from build123d import *

# Parameters (mm, degrees)
BOSS_EXTRU_1_DEPTH         = 3
BOSS_EXTRU_2_DEPTH         = 100
R_P_TITION_LIN_AIRE1_COUNT = 2
R_P_TITION_LIN_AIRE1_PITCH = 103
ESQUISSE5_W                = 2.97567345
ESQUISSE5_H                = 100
BOSS_EXTRU_3_DEPTH         = 47
ESQUISSE6_W                = 2.99565123
ESQUISSE6_H                = 100
ENL_V_MAT_EXTRU_1_REACH    = 125.839
ESQUISSE7_W                = 30
ESQUISSE7_H                = 20
ESQUISSE9_R                = 1.462141601
ENL_V_MAT_EXTRU_8_DEPTH    = 10


with BuildPart() as part:
    # Esquisse2 → Boss.-Extru.1 (new body)
    with BuildSketch(Plane.XY):
        Polygon((0, 0), (0, 50), (3.942801894, 50), (37.89429856, 28.942702884), (30, 0), align=None)
    boss_extru_1 = extrude(amount=BOSS_EXTRU_1_DEPTH)

    # Esquisse4 → Boss.-Extru.2 (add)
    with BuildSketch(Plane.XY.offset(3)):
        Polygon((0, 0), (0, 3.006117571), (30.819936884, 3.006117571), (30, 0), align=None)
    extrude(amount=BOSS_EXTRU_2_DEPTH)

    # Répétition linéaire1: Boss.-Extru.1 ×2
    with Locations(*[(0, 0, i * R_P_TITION_LIN_AIRE1_PITCH) for i in range(1, R_P_TITION_LIN_AIRE1_COUNT)]):
        add(boss_extru_1)

    # Esquisse5 → Boss.-Extru.3 (add)
    with BuildSketch(Plane(origin=(0, 3.006117571, 0), x_dir=(1, 0, 0), z_dir=(0, 1, 0))):
        with Locations((1.487836725, -53)):
            Rectangle(ESQUISSE5_W, ESQUISSE5_H)
    extrude(amount=BOSS_EXTRU_3_DEPTH)

    # Balayage1: sweep along a curve in space
    with BuildLine() as balayage1_path:
        Line((30.819936884, 3.006117571, 103), (37.89429856, 28.942702884, 103))
    # Esquisse6 → Balayage1 (sweep)
    with BuildSketch(Plane(origin=(0, 3.006117571, 0), x_dir=(1, 0, 0), z_dir=(0, 1, 0))):
        with Locations((29.322111269, -53)):
            Rectangle(ESQUISSE6_W, ESQUISSE6_H)
    sweep(path=balayage1_path.line)

    # Esquisse7 → Enlèv. mat.-Extru.1 (cut, up to next)
    with BuildSketch(Plane(origin=(27.922668341, -7.616077924, 0), x_dir=(0, 0, -1), z_dir=(0.9647567628041306, -0.2631432853479158, 0)), mode=Mode.PRIVATE) as enl_v_mat_extru_1_sk1:
        with Locations((-78, 22.89429856)):
            Rectangle(ESQUISSE7_W, ESQUISSE7_H)
    enl_v_mat_extru_1_tool1 = extrude(enl_v_mat_extru_1_sk1.sketch, amount=-ENL_V_MAT_EXTRU_1_REACH, mode=Mode.PRIVATE) & part.part
    enl_v_mat_extru_1 = enl_v_mat_extru_1_tool1.solids().sort_by_distance((33.947149, 14.471351, 78))[0]
    add(enl_v_mat_extru_1, mode=Mode.SUBTRACT)

    # Symétrie1: Enlèv. mat.-Extru.1 across plane
    add(enl_v_mat_extru_1.mirror(Plane.XY.offset(53)), mode=Mode.SUBTRACT)

    # Esquisse9 → Enlèv. mat.-Extru.8 (cut)
    with BuildSketch(Plane(origin=(2.97567345, 0, 0), x_dir=(0, 0, -1), z_dir=(1, 0, 0))):
        with Locations((-84.107906361, 18.157522719)):
            Circle(ESQUISSE9_R)
    enl_v_mat_extru_8 = extrude(amount=-ENL_V_MAT_EXTRU_8_DEPTH, mode=Mode.SUBTRACT)

    # Symétrie3: Enlèv. mat.-Extru.8 across plane
    add(enl_v_mat_extru_8.mirror(Plane.XY.offset(53)), mode=Mode.SUBTRACT)


solid = part.part
The model under review builds one solid part; all positions refer to its coordinate system, in mm. A direction names the side the tool comes from. Coordinates: 2 decimals unless noted, no trailing zeros. Order: outer loops, then holes, each group sorted by start corner. A loop starts at its lowest first (then second) coordinate and runs counter-clockwise, first axis right, second up. Notation, with made-up numbers: (-40, 44) -> (-12, 44) arc R8 ccw to (-12, 49) -> close; hole circle Ø10 at (17, -12.75). An arc over 180 degrees is marked (long way). Answer in a Markdown table with one row per item.
(1) Wall thickness on line 1 along Z through (x, y) = (29, 5.5); line 2 along Z through (x, y) = (28.5, 17); line 3 along Y through (x, z) = (24, 11.5): over which ranges is each line inside the solid? List them lowest first.
Answers:
| item | result |
|---|---|
| line 1 | 0 to 13, 43 to 63, 93 to 106 |
| line 2 | 0 to 3, 103 to 106 |
| line 3 | 0 to 3.01 |
(2) Consider section D-D (x = 7.5). Write out the cut boundary in (y, z), plus the area to 3 significant figures.
Answers:
| item | result |
|---|---|
| outline | (0, 0) -> (47.79, 0) -> (47.79, 3) -> (3.01, 3) -> (3.01, 103) -> (47.79, 103) -> (47.79, 106) -> (0, 106) -> close |
| area | 587 mm² |
(3) Consider section A-A (z = 88). Write out the cut boundary in (x, y).
Answers:
| item | result |
|---|---|
| outline | (0, 0) -> (30, 0) -> (31.32, 4.82) -> (28.53, 5.58) -> (27.82, 3.01) -> (2.98, 3.01) -> (2.98, 50.01) -> (0, 50.01) -> close; (33.79, 24.88) -> (36.58, 24.12) -> (37.89, 28.94) -> (34.9, 28.94) -> close |
(4) The part is to be moulded in two halves that separate along X. For faces 1 (the flat face through (35.204, 24.494, 78.21)), 2 (the flat face through (15, 20, 0)), 3 (the flat face through (29.94, 5.2, 78.21)), say which applies: +X half, -X half, draft (parallel to the pull), parting line (faces both ways), or undercut.
Answers:
| item | result |
|---|---|
| face 1 | undercut |
| face 2 | draft |
| face 3 | +X half |
(5) Consider section B-B (y = 21). Write out the cut boundary in (x, z), plus the area to 3 significant figures.
Answers:
| item | result |
|---|---|
| outline | (0, 0) -> (35.73, 0) -> (35.73, 13) -> (32.73, 13) -> (32.73, 3) -> (2.98, 3) -> (2.98, 103) -> (32.73, 103) -> (32.73, 93) -> (35.73, 93) -> (35.73, 106) -> (0, 106) -> close; (32.73, 43) -> (35.73, 43) -> (35.73, 63) -> (32.73, 63) -> close |
| area | 632 mm² |
(6) Machinability: for faces 4 (the flat face through (31.411, 16.156, 52.3)), 5 (the flat face through (35.204, 24.494, 27.79)), 6 (the flat face through (29.94, 5.2, 27.79)), which of the approach directions +Z, -Z, +X, -X, +Y, -Y give a long, thin tool a straight path to every point of the face, cutting with its end or side? Answer none if there is none.
Answers:
| item | result |
|---|---|
| face 4 | +Y |
| face 5 | -Y |
| face 6 | +X, +Y |
(7) Consider section C-C (z = 22). Write out the cut boundary in (x, y), plus the area to 3 significant figures.
Answers:
| item | result |
|---|---|
| outline | (0, 0) -> (30, 0) -> (31.32, 4.82) -> (28.53, 5.58) -> (27.82, 3.01) -> (2.98, 3.01) -> (2.98, 16.7) -> (0, 16.7) -> close; (0, 19.62) -> (2.98, 19.62) -> (2.98, 50.01) -> (0, 50.01) -> close; (33.79, 24.88) -> (36.58, 24.12) -> (37.89, 28.94) -> (34.9, 28.94) -> close |
| area | 242 mm² |
(8) Insertion check: pin 1 (0.9 mm diameter, centred on x = 3, z = 1, fed in from +Y); pin 2 (20 mm diameter, centred on x = 17.5, z = 76, fed in from +Y); pin 3 (8 mm diameter, centred on y = 24.5, z = 27, fed in from +X); pin 4 (1 mm diameter, centred on x = 22.5, y = 41, fed in from +Z). Each pin has a flat end and moves straight along its axis. Give the tip position at first contact, or say it passes through.
Answers:
| item | result |
|---|---|
| pin 1 | y = 50 |
| pin 2 | y = 3.01 |
| pin 3 | x = 37.77 |
| pin 4 | through |
